Verification items for this drawing (mm, ordinates from the low corner). Coordinates: 2 decimals unless noted, no trailing zeros. Write each loop counter-clockwise with the first axis right and the second up, starting at its lowest first coordinate (ties: lowest second). Pieces come first, ordered by that corner, then holes. Notation, with made-up numbers: (26.25, 82) -> (69.25, 82) arc R12 cw to (69.25, 98) -> close; hole circle Ø3 at (21.25, 22.5). An arc over 180 degrees is marked (long way). Answer as CSV lines item,"result".
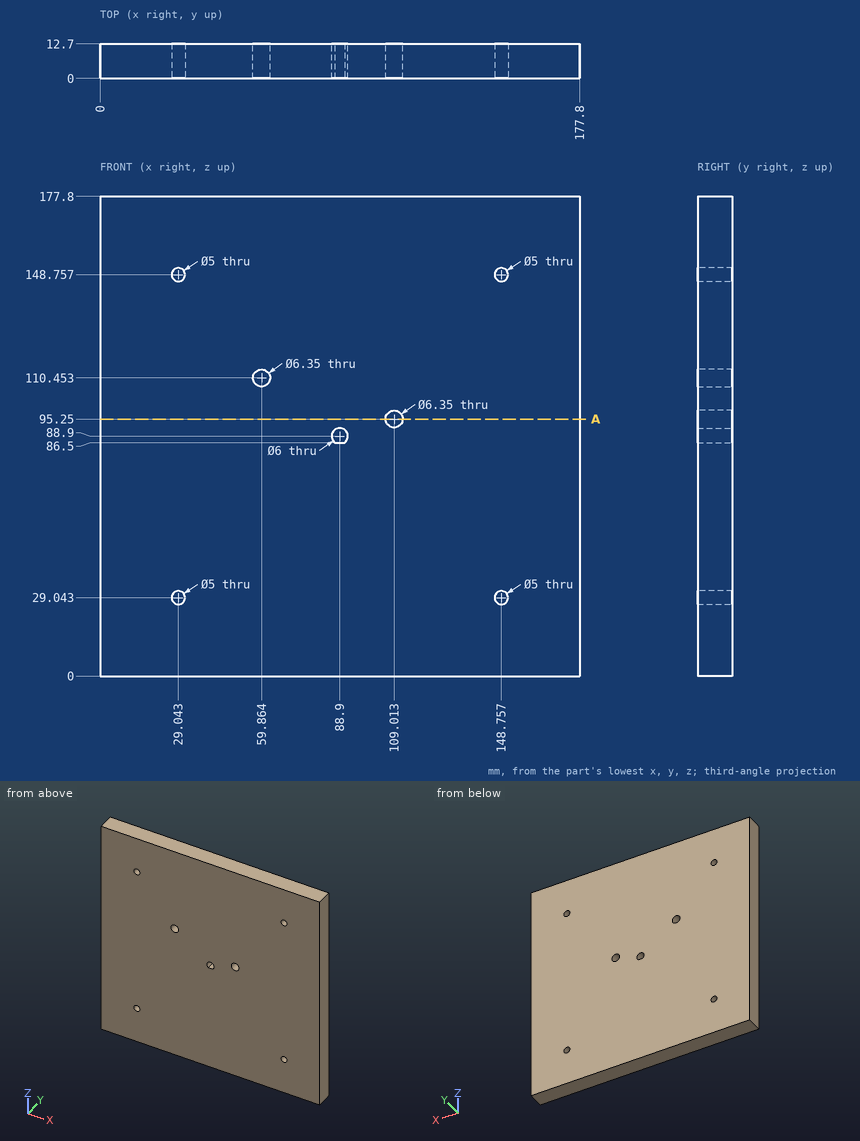
Item 1: Thickness scan on probe 1 along X at (y, z) = (7.25, 88.9); probe 2 along Z at (x, y) = (87, 4.5); probe 3 along Z at (x, y) = (111, 2) (1 decimal). Record the ranges inside material, lowest first.
Responses:
probe 1,"x = 0 to 85.9, 91.9 to 177.8"
probe 2,"z = 0 to 86.58, 91.22 to 177.8"
probe 3,"z = 0 to 92.8, 97.7 to 177.8"
Item 2: Depth check by flat-ended pin: pin 1 Ø12 at (x, z) = (73, 49) entering from -Y. Enter the tip coordinate at first touch or a pass-through.
Responses:
pin 1,"stops at y = 0"
Item 3: Cross-section at A-A, the plane z = 95.25. Record the cut outline in (x, y), plus the area to 3 significant figures.
Responses:
outline,"(0, 0) -> (105.84, 0) -> (105.84, 12.7) -> (0, 12.7) -> close; (112.19, 0) -> (177.8, 0) -> (177.8, 12.7) -> (112.19, 12.7) -> close"
area,"2,180 mm2"
